from build123d import *

# Parameters (mm, degrees)
F0_W     = 160
F0_H     = 85.483871
F1_DEPTH = 20
F0_H_2   = 4.516129
F2_DEPTH = 12
F3_W     = 160
F3_H     = 4
F4_DEPTH = 8


with BuildPart() as f1:
    # F0 (on Front) → F1 (new body)
    with BuildSketch(Plane.XZ):
        with Locations((11.642713, 9.040126)):
            Rectangle(F0_W, F0_H)
    extrude(amount=F1_DEPTH)

    # F0 (on Front) → F2 (join)
    with BuildSketch(Plane.XZ):
        with Locations((11.642713, -35.959874)):
            Rectangle(F0_W, F0_H_2)
    extrude(amount=F2_DEPTH)

    # F3 (on face) → F4 (cut)
    with BuildSketch(Plane.XZ.offset(20)):
        with Locations((11.642713, 41.782062)):
            Rectangle(F3_W, F3_H)
    extrude(amount=-F4_DEPTH, mode=Mode.SUBTRACT)


solid = f1.part
Could you check a few things on this model? Use its own coordinates, in mm. A direction names the side the tool comes from. Coordinates: 2 decimals unless noted, no trailing zeros. Loops run counter-clockwise (first coordinate to the right, second up) from the corner with the lowest first, then second, coordinate; pieces in that order, holes last. Notation, with made-up numbers: (78, 77.5) -> (135, 77.5) arc R22 ccw to (135, 83.5) -> close; hole circle Ø10 at (-7.5, 3.25). An arc over 180 degrees is marked (long way). Answer in a Markdown table with one row per item.
(1) Imagine slicing it at A-A (y = -17.75). List the corners of the cut face in (x, z) for me.
Results found:
| item | result |
|---|---|
| outline | (-68.36, -33.7) -> (91.64, -33.7) -> (91.64, 39.78) -> (-68.36, 39.78) -> close; (-68.36, 43.78) -> (91.64, 43.78) -> (91.64, 51.78) -> (-68.36, 51.78) -> close |
(2) Imagine slicing it at B-B (x = 29.5). List the corners of the cut face in (y, z) for me.
Results found:
| item | result |
|---|---|
| outline | (-20, -33.7) -> (-12, -33.7) -> (-12, -38.22) -> (0, -38.22) -> (0, 51.78) -> (-20, 51.78) -> (-20, 43.78) -> (-12, 43.78) -> (-12, 39.78) -> (-20, 39.78) -> close |
(3) Thinking about a two-plate mould opening in Z: for faces 1 (the face through (11, -10, 51.782)), 2 (the face through (-68.357, -10, 6)), 3 (the face through (11, -12, 42)), 4 (the face through (11, -16, 43.782)), which applies, released by +Z, released by -Z, zero draft, split by the parting line, or undercut?
Results found:
| item | result |
|---|---|
| face 1 | released by +Z |
| face 2 | zero draft |
| face 3 | undercut |
| face 4 | undercut |
(4) For faces 5 (the face through (11, -20, 4)), 6 (the face through (11, -12, -36)), 7 (the face through (11, -16, 39.782)), which set-ups out of +Z, -Z, +X, -X, +Y, -Y let a thin tool reach every point of the face, with its end or its side?
Results found:
| item | result |
|---|---|
| face 5 | +Z, -Z, +X, -X, -Y |
| face 6 | -Z, +X, -X, -Y |
| face 7 | +X, -X, -Y |
(5) If I drill on probe 1 along Z at (x, y) = (47, -18.25); probe 2 along Y at (x, z) = (-22, 41), over which ranges is the centre line in solid material (lowest first)?
Results found:
| item | result |
|---|---|
| probe 1 | z = -33.7 to 39.78, 43.78 to 51.78 |
| probe 2 | y = -12 to 0 |
(6) Will these pins go through, and if not, where does the flat tip stop? pin 1 Ø2.5 at (x, z) = (-24, -35.5) entering from -Y; pin 2 Ø6 at (x, z) = (60, -8) entering from +Y; pin 3 Ø4 at (x, y) = (21.5, -15) entering from -Z.
Results found:
| item | result |
|---|---|
| pin 1 | stops at y = -12 |
| pin 2 | stops at y = 0 |
| pin 3 | stops at z = -33.7 |
